```python
from build123d import *

# Parameters (mm, degrees)
SKETCH1_W           = 812.8
SKETCH1_H           = 457.2
BOSS_EXTRUDE1_DEPTH = 6.35
SKETCH3_R           = 35
SKETCH3_R_2         = 3.175
SKETCH3_R_3         = 6.35
CUT_EXTRUDE1_DEPTH  = 6.35


with BuildPart() as part:
    # Sketch1 → Boss-Extrude1 (new body)
    with BuildSketch(Plane(origin=(0, 0, 0), x_dir=(1, 0, 0), z_dir=(0, 1, 0))):
        with Locations((-36.138533541, -41.56723869)):
            Rectangle(SKETCH1_W, SKETCH1_H)
    extrude(amount=BOSS_EXTRUDE1_DEPTH)

    # Sketch3 → Cut-Extrude1 (cut)
    with BuildSketch(Plane(origin=(0, 6.35, 0), x_dir=(1, 0, 0), z_dir=(0, 1, 0))):
        with Locations((-239.338533541, 129.88276131)):
            Circle(SKETCH3_R)
        with Locations((-125.038533541, 129.88276131)):
            Circle(SKETCH3_R)
        with Locations((-10.738533541, 129.88276131)):
            Circle(SKETCH3_R)
        with Locations((103.561466459, 129.88276131)):
            Circle(SKETCH3_R)
        with Locations((217.861466459, 129.88276131)):
            Circle(SKETCH3_R)
        with Locations((-125.038533541, 15.58276131)):
            Circle(SKETCH3_R)
        with Locations((-10.738533541, 15.58276131)):
            Circle(SKETCH3_R)
        with Locations((103.561466459, 15.58276131)):
            Circle(SKETCH3_R)
        with Locations((217.861466459, 15.58276131)):
            Circle(SKETCH3_R)
        with Locations((-239.338533541, 15.58276131)):
            Circle(SKETCH3_R)
        with Locations((-391.738533541, 142.58276131)):
            Circle(SKETCH3_R_2)
        with Locations((-372.688533541, 142.58276131)):
            Circle(SKETCH3_R_2)
        with Locations((-372.688533541, 104.48276131)):
            Circle(SKETCH3_R_2)
        with Locations((-372.688533541, 66.38276131)):
            Circle(SKETCH3_R_2)
        with Locations((-372.688533541, 28.28276131)):
            Circle(SKETCH3_R_2)
        with Locations((-372.688533541, -9.81723869)):
            Circle(SKETCH3_R_2)
        with Locations((-372.688533541, -47.91723869)):
            Circle(SKETCH3_R_2)
        with Locations((-372.688533541, -86.01723869)):
            Circle(SKETCH3_R_2)
        with Locations((-372.688533541, -124.11723869)):
            Circle(SKETCH3_R_2)
        with Locations((-372.688533541, -162.21723869)):
            Circle(SKETCH3_R_2)
        with Locations((-372.688533541, -200.31723869)):
            Circle(SKETCH3_R_2)
        with Locations((-391.738533541, 104.48276131)):
            Circle(SKETCH3_R_2)
        with Locations((-391.738533541, 66.38276131)):
            Circle(SKETCH3_R_2)
        with Locations((-391.738533541, 28.28276131)):
            Circle(SKETCH3_R_2)
        with Locations((-391.738533541, -9.81723869)):
            Circle(SKETCH3_R_2)
        with Locations((-391.738533541, -47.91723869)):
            Circle(SKETCH3_R_2)
        with Locations((-391.738533541, -86.01723869)):
            Circle(SKETCH3_R_2)
        with Locations((-391.738533541, -124.11723869)):
            Circle(SKETCH3_R_2)
        with Locations((-391.738533541, -162.21723869)):
            Circle(SKETCH3_R_2)
        with Locations((-391.738533541, -200.31723869)):
            Circle(SKETCH3_R_2)
        with Locations((-429.838533541, 174.33276131)):
            Circle(SKETCH3_R_3)
        with Locations((-429.838533541, -257.46723869)):
            Circle(SKETCH3_R_3)
        with Locations((357.561466459, -257.46723869)):
            Circle(SKETCH3_R_3)
        with Locations((357.561466459, 174.33276131)):
            Circle(SKETCH3_R_3)
        with Locations((-266.770533541, 167.42276131)):
            Circle(SKETCH3_R_2)
        with Locations((-273.775133316, 160.418161536)):
            Circle(SKETCH3_R_2)
        with Locations((-152.470533541, 167.42276131)):
            Circle(SKETCH3_R_2)
        with Locations((-159.475133316, 160.418161536)):
            Circle(SKETCH3_R_2)
        with Locations((-38.170533541, 167.42276131)):
            Circle(SKETCH3_R_2)
        with Locations((-45.175133316, 160.418161536)):
            Circle(SKETCH3_R_2)
        with Locations((76.129466459, 167.42276131)):
            Circle(SKETCH3_R_2)
        with Locations((69.124866684, 160.418161536)):
            Circle(SKETCH3_R_2)
        with Locations((190.429466459, 167.42276131)):
            Circle(SKETCH3_R_2)
        with Locations((183.424866684, 160.418161536)):
            Circle(SKETCH3_R_2)
        with Locations((190.429466459, -21.95723869)):
            Circle(SKETCH3_R_2)
        with Locations((76.129466459, -21.95723869)):
            Circle(SKETCH3_R_2)
        with Locations((69.124866684, -14.952638915)):
            Circle(SKETCH3_R_2)
        with Locations((183.424866684, -14.952638915)):
            Circle(SKETCH3_R_2)
        with Locations((-38.170533541, -21.95723869)):
            Circle(SKETCH3_R_2)
        with Locations((-45.175133316, -14.952638915)):
            Circle(SKETCH3_R_2)
        with Locations((-152.470533541, -21.95723869)):
            Circle(SKETCH3_R_2)
        with Locations((-159.475133316, -14.952638915)):
            Circle(SKETCH3_R_2)
        with Locations((-266.770533541, -21.95723869)):
            Circle(SKETCH3_R_2)
        with Locations((-273.775133316, -14.952638915)):
            Circle(SKETCH3_R_2)
        with Locations((-273.775133316, -68.181838464)):
            Circle(SKETCH3_R_2)
        with Locations((-266.770533541, -61.17723869)):
            Circle(SKETCH3_R_2)
        with Locations((-159.475133316, -68.181838464)):
            Circle(SKETCH3_R_2)
        with Locations((-152.470533541, -61.17723869)):
            Circle(SKETCH3_R_2)
        with Locations((-45.175133316, -68.181838464)):
            Circle(SKETCH3_R_2)
        with Locations((-38.170533541, -61.17723869)):
            Circle(SKETCH3_R_2)
        with Locations((183.424866684, -68.181838464)):
            Circle(SKETCH3_R_2)
        with Locations((69.124866684, -68.181838464)):
            Circle(SKETCH3_R_2)
        with Locations((76.129466459, -61.17723869)):
            Circle(SKETCH3_R_2)
        with Locations((190.429466459, -61.17723869)):
            Circle(SKETCH3_R_2)
        with Locations((183.424866684, -243.552638915)):
            Circle(SKETCH3_R_2)
        with Locations((190.429466459, -250.55723869)):
            Circle(SKETCH3_R_2)
        with Locations((69.124866684, -243.552638915)):
            Circle(SKETCH3_R_2)
        with Locations((76.129466459, -250.55723869)):
            Circle(SKETCH3_R_2)
        with Locations((-45.175133316, -243.552638915)):
            Circle(SKETCH3_R_2)
        with Locations((-38.170533541, -250.55723869)):
            Circle(SKETCH3_R_2)
        with Locations((-159.475133316, -243.552638915)):
            Circle(SKETCH3_R_2)
        with Locations((-152.470533541, -250.55723869)):
            Circle(SKETCH3_R_2)
        with Locations((-273.775133316, -243.552638915)):
            Circle(SKETCH3_R_2)
        with Locations((-266.770533541, -250.55723869)):
            Circle(SKETCH3_R_2)
        with Locations((-239.338533541, -98.71723869)):
            Circle(SKETCH3_R)
        with Locations((217.861466459, -98.71723869)):
            Circle(SKETCH3_R)
        with Locations((103.561466459, -98.71723869)):
            Circle(SKETCH3_R)
        with Locations((-10.738533541, -98.71723869)):
            Circle(SKETCH3_R)
        with Locations((-125.038533541, -98.71723869)):
            Circle(SKETCH3_R)
        with Locations((217.861466459, -213.01723869)):
            Circle(SKETCH3_R)
        with Locations((103.561466459, -213.01723869)):
            Circle(SKETCH3_R)
        with Locations((-10.738533541, -213.01723869)):
            Circle(SKETCH3_R)
        with Locations((-125.038533541, -213.01723869)):
            Circle(SKETCH3_R)
        with Locations((-239.338533541, -213.01723869)):
            Circle(SKETCH3_R)
    extrude(amount=-CUT_EXTRUDE1_DEPTH, mode=Mode.SUBTRACT)


solid = part.part
```
Here's how the part is built. I have some questions about the finished solid (model axes, mm). Give positions to 0.01 mm unless a question says otherwise; leave off trailing zeros. Loops run counter-clockwise (first coordinate to the right, second up) from the corner with the lowest first, then second, coordinate; pieces in that order, holes last. Notation, with made-up numbers: (-13.5, 53) -> (35.5, 53) arc R12 cw to (35.5, 59) -> close; hole circle Ø11 at (-2.75, 61.25). An arc over 180 degrees is marked (long way). Use one line per item in the form item = value. Start each with the question number.
1) Imagine slicing it at B-B (y = 3.75). Count the separate pieces of the cut face and the enclosed holes in it, then the cut area to 3 significant figures.
2) Please list where these lines run through material, in increasing order: line 1 along Z through (x, y) = (215, 0.5); line 2 along X through (y, z) = (0.75, -129); line 3 along X through (y, z) = (4, -167).
3) Thinking about a two-plate mould opening in Z: for faces 1 (the face through (95.974, 3.219, 247.185)), 2 (the face through (-18.326, 3.219, 247.185)), 3 (the face through (-42, 0, 38)), which applies, +Z half, -Z half, draft (parallel to the pull), parting line (faces both ways), or undercut?
4) Imagine slicing it at C-C (x = -224.5). Please give me the cut outline in (y, z).
5) Imagine slicing it at A-A (x = 128.5). Please give me the cut outline in (y, z), then the cut area to 3 significant figures.
6) For P1, Ø5.5, axis at x = 183.42, z = 243.55, coming from the -Y side, with a flat end and sliding along its axis, tell me the tip position at first contact or that it passes through.
Check values:
q1.separate_pieces = 1
q1.enclosed_holes = 84
q1.area = 292,000 mm^2
q2.line_1 = -187.03 to -164.77, -95 to -50.47, 19.3 to 63.83, 133.6 to 178.13, 247.9 to 270.17
q2.line_2 = -442.54 to -274.33, -204.35 to -160.03, -90.05 to -45.73, 24.25 to 68.57, 138.55 to 182.87, 252.85 to 370.26
q2.line_3 = -442.54 to -269.92, -263.62 to -155.62, -149.32 to -41.32, -35.02 to 72.98, 79.28 to 187.28, 193.58 to 370.26
q3.face_1 = undercut
q3.face_2 = undercut
q3.face_3 = draft
q4.outline = (0, -187.03) -> (6.35, -187.03) -> (6.35, -161.58) -> (0, -161.58) -> close; (0, -98.18) -> (6.35, -98.18) -> (6.35, -47.28) -> (0, -47.28) -> close; (0, 16.12) -> (6.35, 16.12) -> (6.35, 67.02) -> (0, 67.02) -> close; (0, 130.42) -> (6.35, 130.42) -> (6.35, 181.32) -> (0, 181.32) -> close; (0, 244.72) -> (6.35, 244.72) -> (6.35, 270.17) -> (0, 270.17) -> close
q5.outline = (0, -187.03) -> (6.35, -187.03) -> (6.35, -154.44) -> (0, -154.44) -> close; (0, -105.33) -> (6.35, -105.33) -> (6.35, -40.14) -> (0, -40.14) -> close; (0, 8.97) -> (6.35, 8.97) -> (6.35, 74.16) -> (0, 74.16) -> close; (0, 123.27) -> (6.35, 123.27) -> (6.35, 188.46) -> (0, 188.46) -> close; (0, 237.57) -> (6.35, 237.57) -> (6.35, 270.17) -> (0, 270.17) -> close
q5.area = 1,660 mm^2
q6.P1 = through
